```python
from build123d import *

# Parameters (mm, degrees)
F4_DEPTH = 4
F2_R     = 1.5
F5_DEPTH = 25


with BuildPart() as f4:
    # F3 (on Top) → F4 (new body)
    with BuildSketch(Plane.XY):
        with BuildLine():
            Line((-126.9926666777, -4.22592549), (-132.5, 0))
            Line((-132.5, 0), (-135.7426666777, -4.22592549))
            Line((-135.7426666777, -4.22592549), (-139.4059428918, -9))
            Line((-139.4059428918, -9), (-132.4324272279, -35.0255147652))
            ThreePointArc((-132.4324272279, -35.0255147652), (-130.5316607318, -39.6787820716), (-127.530710333, -43.7111643205))
            Line((-127.530710333, -43.7111643205), (-128.7537766971, -42.4391498951))
            ThreePointArc((-128.7537766971, -42.4391498951), (-125.7528262983, -46.4715321441), (-123.8520598023, -51.1247994505))
            Line((-123.8520598023, -51.1247994505), (-112.6451262464, -92.9496448783))
            ThreePointArc((-112.6451262464, -92.9496448783), (-111.0012337894, -103.4455930684), (-111.6119870301, -114.0519256721))
            Line((-111.6119870301, -114.0519256721), (-113.4985999884, -125.4551601363))
            ThreePointArc((-113.4985999884, -125.4551601363), (-100.9391467421, -112.7279601319), (-84.7430925287, -120.3048535396))
            Line((-84.7430925287, -120.3048535396), (-93.2455614317, -105.4002627224))
            ThreePointArc((-93.2455614317, -105.4002627224), (-96.0587011908, -99.6394303241), (-98.1115817937, -93.5659941915))
            Line((-98.1115817937, -93.5659941915), (-120.7709716444, -9))
            Line((-120.7709716444, -9), (-126.9926666777, -4.22592549))
        make_face()
        with BuildLine():
            ThreePointArc((-82.7064765239, -127.9851719833), (-83.2242795567, -124.0122921667), (-84.7430925287, -120.3048535396))
            ThreePointArc((-84.7430925287, -120.3048535396), (-100.9391467421, -112.7279601319), (-113.4985999884, -125.4551601363))
            ThreePointArc((-113.4985999884, -125.4551601363), (-99.4757452701, -143.4331154338), (-82.7064765239, -127.9851719833))
        make_face()
    extrude(amount=F4_DEPTH)

    # F0 (on Top) + F1 (on Top) + F2 (on Top) → F5 (cut)
    with BuildSketch(Plane.XY):
        with BuildLine():
            ThreePointArc((-101.5723892492, -135.2794656723), (-101.4225386155, -134.1412371047), (-102.1214273549, -133.2304275666))
            ThreePointArc((-102.1214273549, -133.2304275666), (-103.2596559226, -133.0805769329), (-104.1704654606, -133.7794656723))
            Line((-104.1704654606, -133.7794656723), (-104.9204654606, -135.078503778))
            ThreePointArc((-104.9204654606, -135.078503778), (-105.0703160943, -136.2167323456), (-104.3714273549, -137.1275418837))
            ThreePointArc((-104.3714273549, -137.1275418837), (-103.2331987872, -137.2773925174), (-102.3223892492, -136.578503778))
            Line((-102.3223892492, -136.578503778), (-101.5723892492, -135.2794656723))
        make_face()
        with BuildLine():
            ThreePointArc((-94.7423749088, -129.9851719833), (-94.3427732188, -129.0204481637), (-94.2064765239, -127.9851719833))
            ThreePointArc((-94.2064765239, -127.9851719833), (-102.0701798291, -126.9498958029), (-94.7423749088, -129.9851719833))
        make_face()
        with BuildLine():
            Line((-107.4647591496, -123.4853497167), (-106.1657210439, -124.2353497167))
            ThreePointArc((-106.1657210439, -124.2353497167), (-105.0274924763, -124.3852003505), (-104.1166829382, -123.6863116111))
            ThreePointArc((-104.1166829382, -123.6863116111), (-103.9668323045, -122.5480830434), (-104.6657210439, -121.6372735054))
            Line((-104.6657210439, -121.6372735054), (-105.9647591496, -120.8872735054))
            ThreePointArc((-105.9647591496, -120.8872735054), (-107.1029877172, -120.7374228716), (-108.0137972553, -121.4363116111))
            ThreePointArc((-108.0137972553, -121.4363116111), (-108.163647889, -122.5745401787), (-107.4647591496, -123.4853497167))
        make_face()
        with BuildLine():
            Line((-92.523528877, -121.142017922), (-91.773528877, -119.8429798164))
            ThreePointArc((-91.773528877, -119.8429798164), (-91.6236782432, -118.7047512487), (-92.3225669827, -117.7939417107))
            ThreePointArc((-92.3225669827, -117.7939417107), (-93.4607955503, -117.6440910769), (-94.3716050883, -118.3429798164))
            Line((-94.3716050883, -118.3429798164), (-95.1216050883, -119.642017922))
            ThreePointArc((-95.1216050883, -119.642017922), (-95.2714557221, -120.7802464897), (-94.5725669827, -121.6910560277))
            ThreePointArc((-94.5725669827, -121.6910560277), (-93.434338415, -121.8409066615), (-92.523528877, -121.142017922))
        make_face()
        with BuildLine():
            ThreePointArc((-90.5282732936, -130.6861338776), (-91.6665018613, -130.5362832439), (-92.5773113993, -131.2351719833))
            ThreePointArc((-92.5773113993, -131.2351719833), (-92.7271620331, -132.373400551), (-92.0282732936, -133.284210089))
            Line((-92.0282732936, -133.284210089), (-90.729235188, -134.034210089))
            ThreePointArc((-90.729235188, -134.034210089), (-89.5910066203, -134.1840607227), (-88.6801970823, -133.4851719833))
            ThreePointArc((-88.6801970823, -133.4851719833), (-88.5303464485, -132.3469434156), (-89.229235188, -131.4361338776))
            Line((-89.229235188, -131.4361338776), (-90.5282732936, -130.6861338776))
        make_face()
    with BuildSketch(Plane.XY):
        with BuildLine():
            ThreePointArc((-123.2354286469, -28.9777747887), (-123.8222865034, -27.7877447782), (-125.1236572146, -27.5288860492))
            Line((-125.1236572146, -27.5288860492), (-124.3472000793, -30.4266635281))
            ThreePointArc((-124.3472000793, -30.4266635281), (-123.5453986365, -29.8909169322), (-123.2354286469, -28.9777747887))
        make_face()
        with BuildLine():
            Line((-124.3472000793, -30.4266635281), (-125.1236572146, -27.5288860492))
            ThreePointArc((-125.1236572146, -27.5288860492), (-126.1843173864, -29.3660033563), (-124.3472000793, -30.4266635281))
        make_face()
        with BuildLine():
            ThreePointArc((-128.7353333554, -8.45185098), (-129.3221912118, -7.2618209696), (-130.623561923, -7.0029622406))
            Line((-130.623561923, -7.0029622406), (-129.8471047877, -9.9007397195))
            ThreePointArc((-129.8471047877, -9.9007397195), (-129.0453033449, -9.3649931235), (-128.7353333554, -8.45185098))
        make_face()
        with BuildLine():
            Line((-129.8471047877, -9.9007397195), (-130.623561923, -7.0029622406))
            ThreePointArc((-130.623561923, -7.0029622406), (-131.6842220948, -8.8400795477), (-129.8471047877, -9.9007397195))
        make_face()
    with BuildSketch(Plane.XY):
        with Locations((-129.6849733529, -21.3822502318)):
            Circle(F2_R)
    extrude(amount=F5_DEPTH, mode=Mode.SUBTRACT)


solid = f4.part
```
Geometry check sheet. Reference: the model listing, model coordinates, mm. A direction names the side the tool comes from. Round coordinates to 2 decimals unless told otherwise and drop trailing zeros. Loops run counter-clockwise (first coordinate to the right, second up) from the corner with the lowest first, then second, coordinate; pieces in that order, holes last. Notation, with made-up numbers: (85, 37.25) - (93, 37.25) arc R23 ccw to (93, 68.25) - close; hole circle Ø9 at (-23, -5.5). An arc over 180 degrees is marked (long way). Write item = value, one per line. Start each with the question number.
1. Thickness scan on line 1 (X direction, y = -123, z = 2.1); line 2 (X direction, y = -9.5, z = 2.4); line 3 (X direction, y = -133.5, z = 2.85). Record the ranges inside material, lowest first.
2. Section check C-C on x = -117.5. Enter the section's corners in (y, z), then the cut area to 3 significant figures.
3. Set-up check for faces 5 (the face through (-112.54, -119.67, 1.97)), 6 (the face through (-88.935, -112.957, 1.972)): record each of +Z, -Z, +X, -X, +Y, -Y from which the full face is reachable in a straight line by a thin tool's end or side.
4. Section check B-B on z = 1.9. Give the number of separate pieces and of enclosed holes in the cut face, then the cut area to 3 significant figures.
5. Mould release check, pull along X, two halves, no side actions. Record for faces 1 (the face through (-96.024, -99.722, 1.972)), 2 (the face through (-125.788, -46.41, 1.972)), 3 (the face through (-128.3, -21.96, 1.97)), 4 (the face through (-111, -77, 4)): released by +X, released by -X, zero draft, split by the parting line, or undercut.
6. Section check A-A on y = -115.5. Enter the section's corners in (x, z), then the cut area to 3 significant figures.
7. Depth check by flat-ended pin: pin 1 (1.5 mm diameter, centred on y = -59, z = 0.5, fed in from -X). Enter the tip coordinate at first touch or a pass-through.
Working result:
q1.line_1 = -113.09 to -107.97, -103.92 to -83.53
q1.line_2 = -139.27 to -131.31, -129.16 to -120.64
q1.line_3 = -112.69 to -103.96, -101.78 to -91.65, -88.69 to -83.72
q2.outline = (-74.83, 0) - (-21.21, 0) - (-21.21, 4) - (-74.83, 4) - close
q2.area = 214 mm^2
q3.face_5 = +Z, -Z, -X
q3.face_6 = +Z, -Z, +X, +Y
q4.separate_pieces = 1
q4.enclosed_holes = 8
q4.area = 2,450 mm^2
q5.face_1 = released by +X
q5.face_2 = released by -X
q5.face_3 = undercut
q5.face_4 = zero draft
q6.outline = (-111.85, 0) - (-87.48, 0) - (-87.48, 4) - (-111.85, 4) - close
q6.area = 97.5 mm^2
q7.pin_1 = -121.94
